```python
from build123d import *

# Parameters (mm, degrees)
SKETCH1_W                                       = 500
SKETCH1_H                                       = 400
BOSS_EXTRUDE1_DEPTH                             = 6.35
CSK_FOR_1_4_FLAT_HEAD_MACHINE_SCREW1_AT_COUNT   = 2
CSK_FOR_1_4_FLAT_HEAD_MACHINE_SCREW1_AT_PITCH   = 127
CSK_FOR_1_4_FLAT_HEAD_MACHINE_SCREW1_2_COUNT    = 2
CSK_FOR_1_4_FLAT_HEAD_MACHINE_SCREW1_2_PITCH    = 219.970452561
CSK_FOR_1_4_FLAT_HEAD_MACHINE_SCREW1_3_COUNT    = 2
CSK_FOR_1_4_FLAT_HEAD_MACHINE_SCREW1_3_PITCH    = 254
CSK_FOR_1_4_FLAT_HEAD_MACHINE_SCREW1_4_COUNT    = 2
CSK_FOR_1_4_FLAT_HEAD_MACHINE_SCREW1_4_PITCH    = 219.970452561
CSK_FOR_1_4_FLAT_HEAD_MACHINE_SCREW1_5_COUNT    = 2
CSK_FOR_1_4_FLAT_HEAD_MACHINE_SCREW1_5_PITCH    = 127
CSK_FOR_10_FLAT_HEAD_MACHINE_SCREW1_D           = 5.1054
CSK_FOR_10_FLAT_HEAD_MACHINE_SCREW1_CSINK_D     = 9.779
CSK_FOR_10_FLAT_HEAD_MACHINE_SCREW1_CSINK_ANGLE = 82
SKETCH12_W                                      = 500
SKETCH12_H                                      = 22.479
CUT_EXTRUDE2_DEPTH                              = 6.35
SKETCH13_W                                      = 500
SKETCH13_H                                      = 22.479
BOSS_EXTRUDE2_DEPTH                             = 6.35
CSK_FOR_10_FLAT_HEAD_MACHINE_SCREW2_D           = 5.1054
CSK_FOR_10_FLAT_HEAD_MACHINE_SCREW2_CSINK_D     = 9.779
CSK_FOR_10_FLAT_HEAD_MACHINE_SCREW2_CSINK_ANGLE = 82
SKETCH22_W                                      = 17.526
SKETCH22_H                                      = 400
CUT_EXTRUDE4_DEPTH                              = 10
FILLET1_R                                       = 12.7
CSK_FOR_1_4_FLAT_HEAD_MACHINE_SCREW2_AT_COUNT   = 2
CSK_FOR_1_4_FLAT_HEAD_MACHINE_SCREW2_AT_PITCH   = 127
CSK_FOR_1_4_FLAT_HEAD_MACHINE_SCREW2_2_COUNT    = 2
CSK_FOR_1_4_FLAT_HEAD_MACHINE_SCREW2_2_PITCH    = 219.970452561
CSK_FOR_1_4_FLAT_HEAD_MACHINE_SCREW2_3_COUNT    = 2
CSK_FOR_1_4_FLAT_HEAD_MACHINE_SCREW2_3_PITCH    = 254
CSK_FOR_1_4_FLAT_HEAD_MACHINE_SCREW2_4_COUNT    = 2
CSK_FOR_1_4_FLAT_HEAD_MACHINE_SCREW2_4_PITCH    = 219.970452561
CSK_FOR_1_4_FLAT_HEAD_MACHINE_SCREW2_5_COUNT    = 2
CSK_FOR_1_4_FLAT_HEAD_MACHINE_SCREW2_5_PITCH    = 127


with BuildPart() as part:
    # Sketch1 → Boss-Extrude1 (new body)
    with BuildSketch(Plane(origin=(0, 0, 0), x_dir=(1, 0, 0), z_dir=(0, 1, 0))):
        with Locations((250, 200)):
            Rectangle(SKETCH1_W, SKETCH1_H)
    extrude(amount=BOSS_EXTRUDE1_DEPTH)

    # Sketch3 → CSK for 1/4 Flat Head Machine Screw1 (revolve, cut)
    with BuildSketch(Plane(origin=(313.5, 6.35, -309.985226281), x_dir=(0, 0, 1), z_dir=(1, 0, 0))):
        Polygon((0, 0), (0, 6.35), (3.3782, 6.35), (3.3782, 4.520932584), (6.4389, 1), (6.4389, 0), align=None)
    csk_for_1_4_flat_head_machine_screw1 = revolve(axis=Axis((313.5, 12.7, -309.985226281), (0, -1, 0)), mode=Mode.SUBTRACT)

    # CSK for 1/4 Flat Head Machine Screw1 at: CSK for 1/4 Flat Head Machine Screw1 ×2
    with Locations(*[(-i * CSK_FOR_1_4_FLAT_HEAD_MACHINE_SCREW1_AT_PITCH, 0, 0) for i in range(1, CSK_FOR_1_4_FLAT_HEAD_MACHINE_SCREW1_AT_COUNT)]):
        add(csk_for_1_4_flat_head_machine_screw1, mode=Mode.SUBTRACT)

    # CSK for 1_4 Flat Head Machine Screw1 2: CSK for 1/4 Flat Head Machine Screw1 ×2
    with Locations(*[Vector(-0.866025403784438, 0, 0.5000000000000012) * (i * CSK_FOR_1_4_FLAT_HEAD_MACHINE_SCREW1_2_PITCH) for i in range(1, CSK_FOR_1_4_FLAT_HEAD_MACHINE_SCREW1_2_COUNT)]):
        add(csk_for_1_4_flat_head_machine_screw1, mode=Mode.SUBTRACT)

    # CSK for 1_4 Flat Head Machine Screw1 3: CSK for 1/4 Flat Head Machine Screw1 ×2
    with Locations(*[Vector(-0.49999999999999767, 0, 0.86602540378444) * (i * CSK_FOR_1_4_FLAT_HEAD_MACHINE_SCREW1_3_PITCH) for i in range(1, CSK_FOR_1_4_FLAT_HEAD_MACHINE_SCREW1_3_COUNT)]):
        add(csk_for_1_4_flat_head_machine_screw1, mode=Mode.SUBTRACT)

    # CSK for 1_4 Flat Head Machine Screw1 4: CSK for 1/4 Flat Head Machine Screw1 ×2
    with Locations(*[(0, 0, i * CSK_FOR_1_4_FLAT_HEAD_MACHINE_SCREW1_4_PITCH) for i in range(1, CSK_FOR_1_4_FLAT_HEAD_MACHINE_SCREW1_4_COUNT)]):
        add(csk_for_1_4_flat_head_machine_screw1, mode=Mode.SUBTRACT)

    # CSK for 1_4 Flat Head Machine Screw1 5: CSK for 1/4 Flat Head Machine Screw1 ×2
    with Locations(*[Vector(0.500000000000001, 0, 0.866025403784438) * (i * CSK_FOR_1_4_FLAT_HEAD_MACHINE_SCREW1_5_PITCH) for i in range(1, CSK_FOR_1_4_FLAT_HEAD_MACHINE_SCREW1_5_COUNT)]):
        add(csk_for_1_4_flat_head_machine_screw1, mode=Mode.SUBTRACT)

    # CSK for #10 Flat Head Machine Screw1 (through all)
    with Locations(Plane(origin=(351.616, 0, -133.475), x_dir=(0, 0, -1), z_dir=(0, -1, 0))):
        with Locations((0, 0), (88, 0), (88, -123.444), (0, -123.444)):
            CounterSinkHole(CSK_FOR_10_FLAT_HEAD_MACHINE_SCREW1_D / 2, CSK_FOR_10_FLAT_HEAD_MACHINE_SCREW1_CSINK_D / 2, counter_sink_angle=CSK_FOR_10_FLAT_HEAD_MACHINE_SCREW1_CSINK_ANGLE)

    # Sketch12 → Cut-Extrude2 (cut)
    with BuildSketch(Plane(origin=(0, 6.35, 0), x_dir=(1, 0, 0), z_dir=(0, 1, 0))):
        with Locations((250, 388.7605)):
            Rectangle(SKETCH12_W, SKETCH12_H)
    extrude(amount=-CUT_EXTRUDE2_DEPTH, mode=Mode.SUBTRACT)

    # Sketch13 → Boss-Extrude2 (add)
    with BuildSketch(Plane(origin=(0, 6.35, 0), x_dir=(1, 0, 0), z_dir=(0, 1, 0))):
        with Locations((250, -11.2395)):
            Rectangle(SKETCH13_W, SKETCH13_H)
    extrude(amount=-BOSS_EXTRUDE2_DEPTH)

    # CSK for #10 Flat Head Machine Screw2 (through all)
    with Locations(Plane(origin=(60.325, 0, -15.621), x_dir=(0, 0, -1), z_dir=(0, -1, 0))):
        with Locations((0, 0), (0, -31.75), (323.8, 0), (323.8, -31.75)):
            CounterSinkHole(CSK_FOR_10_FLAT_HEAD_MACHINE_SCREW2_D / 2, CSK_FOR_10_FLAT_HEAD_MACHINE_SCREW2_CSINK_D / 2, counter_sink_angle=CSK_FOR_10_FLAT_HEAD_MACHINE_SCREW2_CSINK_ANGLE)

    # Sketch22 → Cut-Extrude4 (cut)
    with BuildSketch(Plane(origin=(0, 6.35, 0), x_dir=(1, 0, 0), z_dir=(0, 1, 0))):
        with Locations((491.237, 177.521)):
            Rectangle(SKETCH22_W, SKETCH22_H)
    extrude(amount=-CUT_EXTRUDE4_DEPTH, mode=Mode.SUBTRACT)

    # Fillet1
    fillet1_edges = [part.edges().sort_by_distance(p)[0] for p in [
        (0, 3.175, 22.479),
        (482.474, 3.175, 22.479),
        (482.474, 3.175, -377.521),
        (0, 3.175, -377.521),
    ]]
    fillet(fillet1_edges, radius=FILLET1_R)

    # Sketch28 → CSK for 1/4 Flat Head Machine Screw2 (revolve, cut)
    with BuildSketch(Plane(origin=(249, 6.35, -287.518226281), x_dir=(0, 0, 1), z_dir=(1, 0, 0))):
        Polygon((0, 0), (0, 6.35), (3.3782, 6.35), (3.3782, 3.520932584), (6.4389, 0), align=None)
    csk_for_1_4_flat_head_machine_screw2 = revolve(axis=Axis((249, 12.7, -287.518226281), (0, -1, 0)), mode=Mode.SUBTRACT)

    # CSK for 1/4 Flat Head Machine Screw2 at: CSK for 1/4 Flat Head Machine Screw2 ×2
    with Locations(*[(i * CSK_FOR_1_4_FLAT_HEAD_MACHINE_SCREW2_AT_PITCH, 0, 0) for i in range(1, CSK_FOR_1_4_FLAT_HEAD_MACHINE_SCREW2_AT_COUNT)]):
        add(csk_for_1_4_flat_head_machine_screw2, mode=Mode.SUBTRACT)

    # CSK for 1_4 Flat Head Machine Screw2 2: CSK for 1/4 Flat Head Machine Screw2 ×2
    with Locations(*[Vector(0.8660254037844398, 0, 0.49999999999999795) * (i * CSK_FOR_1_4_FLAT_HEAD_MACHINE_SCREW2_2_PITCH) for i in range(1, CSK_FOR_1_4_FLAT_HEAD_MACHINE_SCREW2_2_COUNT)]):
        add(csk_for_1_4_flat_head_machine_screw2, mode=Mode.SUBTRACT)

    # CSK for 1_4 Flat Head Machine Screw2 3: CSK for 1/4 Flat Head Machine Screw2 ×2
    with Locations(*[Vector(0.5000000000000043, 0, 0.8660254037844363) * (i * CSK_FOR_1_4_FLAT_HEAD_MACHINE_SCREW2_3_PITCH) for i in range(1, CSK_FOR_1_4_FLAT_HEAD_MACHINE_SCREW2_3_COUNT)]):
        add(csk_for_1_4_flat_head_machine_screw2, mode=Mode.SUBTRACT)

    # CSK for 1_4 Flat Head Machine Screw2 4: CSK for 1/4 Flat Head Machine Screw2 ×2
    with Locations(*[(0, 0, i * CSK_FOR_1_4_FLAT_HEAD_MACHINE_SCREW2_4_PITCH) for i in range(1, CSK_FOR_1_4_FLAT_HEAD_MACHINE_SCREW2_4_COUNT)]):
        add(csk_for_1_4_flat_head_machine_screw2, mode=Mode.SUBTRACT)

    # CSK for 1_4 Flat Head Machine Screw2 5: CSK for 1/4 Flat Head Machine Screw2 ×2
    with Locations(*[Vector(-0.4999999999999978, 0, 0.86602540378444) * (i * CSK_FOR_1_4_FLAT_HEAD_MACHINE_SCREW2_5_PITCH) for i in range(1, CSK_FOR_1_4_FLAT_HEAD_MACHINE_SCREW2_5_COUNT)]):
        add(csk_for_1_4_flat_head_machine_screw2, mode=Mode.SUBTRACT)


solid = part.part
```
The listing builds one solid part. Answer for the finished solid, in the listing's coordinates (mm). A direction names the side the tool comes from. Give positions to 0.01 mm unless a question says otherwise; leave off trailing zeros. Write each question's results on one line, items separated by ' | '.
Q1. Straight lines are drawn through the part: probe 1 along X at (y, z) = (1.1, -200); probe 2 along Z at (x, y) = (249, 2.1); probe 3 along X at (y, z) = (5.5, -221.5). For each, find the intervals that lie inside material, in ascending order. Write a range as from..to.
Checked values:
probe 1: x = 0..119.62, 126.38..373.62, 380.38..482.47 | probe 2: z = -377.52..-290.9, -284.14..-70.93, -64.17..22.48 | probe 3: x = 0..225.62, 230.72..349.06, 354.17..482.47
Q2. Each of these flat-tipped pins is pushed along its axis until it touches: P1, Ø11.5, axis at x = 313.5, z = -309.99, coming from the +Y side; P2, Ø3, axis at x = 228.172, z = -133.475, coming from the -Y side; P3, Ø3, axis at x = 342.5, z = -314, coming from the -Y side; P4, Ø11, axis at x = 439.5, z = -177.533, coming from the +Y side. Where does it stop, or does it pass through?
Checked values:
P1: stops at y = 4.56 | P2: passes through | P3: stops at y = 0 | P4: stops at y = 5.27
Q3. Which of the six approach directions +Z, -Z, +X, -X, +Y, -Y give full straight-line access (tool end or side, diameter ignored) to faces 1 (the face through (319.786, 5.857, -91.411)), 2 (the face through (349.251, 2.558, -132.245))?
Checked values:
face 1: +Y | face 2: -Y
Q4. Determine the mould class of faces 3 (the face through (238, 0, -180)), 4 (the face through (310.49, 2.05, -308.07)) for opening direction X: pulls with the +X half, pulls with the -X half, needs draft (parallel to the pull), parting line crosses it, or undercut.
Checked values:
face 3: needs draft | face 4: undercut
